Input: part model. Units: mm. Frame: model coordinates. Face numbers are marked on the shaded views. A direction names the side the tool comes from. Round coordinates to 2 decimals unless told otherwise and drop trailing zeros. Order: outer loops, then holes, each group sorted by start corner. A loop starts at its lowest first (then second) coordinate and runs counter-clockwise, first axis right, second up. Notation, with made-up numbers: (-15, -37) -> (12, -37) arc R35 ccw to (12, 2) -> close; hole circle Ø3 at (75, 63). An arc over 180 degrees is marked (long way). Answer as CSV lines item,"result". Start each with the question number.
1) Section query A-A, the plane z = 0. Output: boundary loops of the cut face in (x, y), and give its area (3 significant figures).
2) Section query B-B, the plane y = 10. Output: boundary loops of the cut face in (x, z), and give its area (3 significant figures).
3) First-contact query: P1, Ø3, axis at y = 12, z = 7.5, coming from the +X side; P2, Ø5, axis at y = 10, z = 7.5, coming from the +X side; P3, Ø10, axis at y = 8.5, z = 5, coming from the +X side; P4, Ø5, axis at x = -3.5, z = -4.5, coming from the -Y side. Flat tips, straight axial feed; report the tip coordinate or a pass-through.
4) Section query C-C, the plane x = -1.5. Output: boundary loops of the cut face in (y, z).
5) Mould query, pull axis Y, two halves, no side actions, for the marked faces 1, 2, 3 and 4. Classes: +Y half, -Y half, draft (parallel to the pull), parting line (faces both ways), or undercut.
6) Line query: L1, parallel to Y at x = 8, z = 7.5; L2, parallel to Y at x = 8.4, z = 0; L3, parallel to Y at x = 0, z = -10.5. Output: solid intervals per line, ascending.
7) Access query for the marked faces 5, 6 and 7. Directions: +Z, -Z, +X, -X, +Y, -Y. A direction counts if a zero-diameter tool reaches every point of the face in a straight line with its end or side. Return the directions, or none.
8) Section query D-D, the plane x = 9.25. Output: boundary loops of the cut face in (y, z).
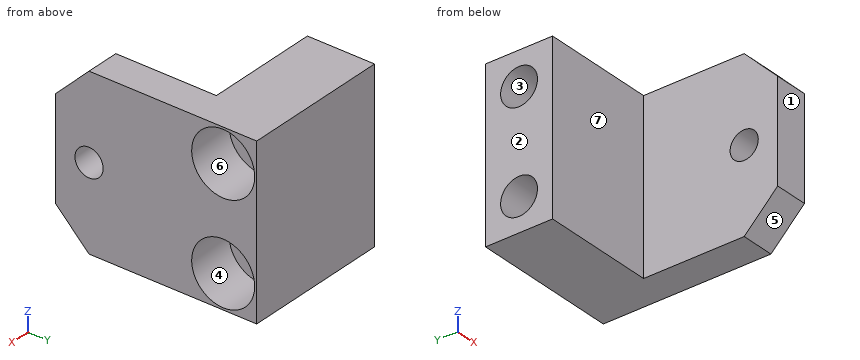
```python
from build123d import *

# Parameters (mm, degrees)
SKETCH_2_W                = 22
SKETCH_2_H                = 30
EXTRUDE_1_DEPTH           = 12.5
SKETCH_3_W                = 17
SKETCH_3_H                = 20
CUT_EXTRUDE_1_DEPTH       = 32.160872902
HOLE_WIZARD_1_D           = 5.5
HOLE_WIZARD_1_CBORE_D     = 9.4
HOLE_WIZARD_1_CBORE_DEPTH = 7
HOLE_WIZARD_M5_1_D        = 4.2
CHAMFER_1_SIZE            = 5


with BuildPart() as part:
    # 草图2 → 凸台-拉伸1 (new, symmetric)
    with BuildSketch(Plane.XY):
        Rectangle(SKETCH_2_W, SKETCH_2_H)
    extrude(amount=EXTRUDE_1_DEPTH, both=True)

    # 草图3 → 切除-拉伸1 (cut, through all)
    with BuildSketch(Plane.XY.offset(12.5)):
        with Locations((-2.5, -5)):
            Rectangle(SKETCH_3_W, SKETCH_3_H)
    extrude(amount=-CUT_EXTRUDE_1_DEPTH, mode=Mode.SUBTRACT)

    # 打孔尺寸根据内六角圆柱头螺钉的类型1 (through all)
    with Locations(Plane(origin=(11, 0, 0), x_dir=(0, 0, -1), z_dir=(1, 0, 0))):
        with Locations((7.5, 10), (-7.5, 10)):
            CounterBoreHole(HOLE_WIZARD_1_D / 2, HOLE_WIZARD_1_CBORE_D / 2, HOLE_WIZARD_1_CBORE_DEPTH)

    # M5 螺纹孔1 (through all)
    with Locations(Plane(origin=(11, 0, 0), x_dir=(0, 0, -1), z_dir=(1, 0, 0))):
        with Locations((0, -10)):
            Hole(HOLE_WIZARD_M5_1_D / 2)

    # 倒角1
    chamfer_1_edges = [part.edges().sort_by_distance(p)[0] for p in [
        (8.5, -15, -12.5),
        (8.5, -15, 12.5),
    ]]
    chamfer(chamfer_1_edges, length=CHAMFER_1_SIZE)


solid = part.part
```
Findings:
1,outline,"(-11, 5) -> (6, 5) -> (6, -7.9) -> (11, -7.9) -> (11, 15) -> (-11, 15) -> close; (6, -15) -> (11, -15) -> (11, -12.1) -> (6, -12.1) -> close"
1,area,"299 mm^2"
2,outline,"(-11, -12.5) -> (11, -12.5) -> (11, -12.2) -> (4, -12.2) -> (4, -10.25) -> (-11, -10.25) -> close; (-11, -4.75) -> (4, -4.75) -> (4, -2.8) -> (11, -2.8) -> (11, 2.8) -> (4, 2.8) -> (4, 4.75) -> (-11, 4.75) -> close; (-11, 10.25) -> (4, 10.25) -> (4, 12.2) -> (11, 12.2) -> (11, 12.5) -> (-11, 12.5) -> close"
2,area,"253 mm^2"
3,P1,"stops at x = 4"
3,P2,"passes through"
3,P3,"stops at x = 11"
3,P4,"stops at y = 5"
4,outline,"(5, -12.5) -> (15, -12.5) -> (15, 12.5) -> (5, 12.5) -> close; hole circle Ø5.5 at (10, -7.5); hole circle Ø5.5 at (10, 7.5)"
5,face 1,"-Y half"
5,face 2,"draft"
5,face 3,"undercut"
5,face 4,"undercut"
6,L1,"y = -15 to 5.3, 14.7 to 15"
6,L2,"y = -15 to -12.1, -7.9 to 15"
6,L3,"y = 5 to 15"
7,face 5,"-Z, +X, -X, -Y"
7,face 6,"+X"
7,face 7,"+Z, -Z, -X, -Y"
8,outline,"(-15, -7.5) -> (-10, -12.5) -> (15, -12.5) -> (15, 12.5) -> (-10, 12.5) -> (-15, 7.5) -> close; hole circle Ø4.2 at (-10, 0); hole circle Ø9.4 at (10, -7.5); hole circle Ø9.4 at (10, 7.5)"
